from build123d import *

# Parameters (mm, degrees)
F0_R     = 1.5
F1_DEPTH = 3
F2_DEPTH = 7
F0_W     = 5
F0_H     = 56.2
F3_DEPTH = 23
F4_R     = 2.1
F5_DEPTH = 5
F6_R     = 5


with BuildPart() as f1:
    # F0 (on Top) → F1 (new body)
    with BuildSketch(Plane.XY):
        with BuildLine():
            Line((-39.5, 28.1), (-41.7, 28.1))
            ThreePointArc((-41.7, 28.1), (-42.4071067812, 27.8071067812), (-42.7, 27.1))
            Line((-42.7, 27.1), (-42.7, -27.1))
            ThreePointArc((-42.7, -27.1), (-42.4071067812, -27.8071067812), (-41.7, -28.1))
            Line((-41.7, -28.1), (-39.5, -28.1))
            Line((-39.5, -28.1), (39.5, -28.1))
            Line((39.5, -28.1), (41.7, -28.1))
            ThreePointArc((41.7, -28.1), (42.4071067812, -27.8071067812), (42.7, -27.1))
            Line((42.7, -27.1), (42.7, 27.1))
            ThreePointArc((42.7, 27.1), (42.4071067812, 27.8071067812), (41.7, 28.1))
            Line((41.7, 28.1), (39.5, 28.1))
            Line((39.5, 28.1), (-39.5, 28.1))
        make_face()
        with BuildLine():
            ThreePointArc((-36.4, -25), (-37.3079689783, -27.1920310217), (-39.5, -28.1))
            ThreePointArc((-39.5, -28.1), (-41.6920310217, -22.8079689783), (-36.4, -25))
        make_face(mode=Mode.SUBTRACT)
        with BuildLine():
            Line((27.5, -17), (-27.5, -17))
            ThreePointArc((-27.5, -17), (-31, -13.5), (-27.5, -10))
            Line((-27.5, -10), (27.5, -10))
            ThreePointArc((27.5, -10), (31, -13.5), (27.5, -17))
        make_face(mode=Mode.SUBTRACT)
        with BuildLine():
            ThreePointArc((42.6, -25), (41.6920310217, -27.1920310217), (39.5, -28.1))
            ThreePointArc((39.5, -28.1), (37.3079689783, -22.8079689783), (42.6, -25))
        make_face(mode=Mode.SUBTRACT)
        with BuildLine():
            ThreePointArc((-27.5, 10), (-31, 13.5), (-27.5, 17))
            Line((-27.5, 17), (27.5, 17))
            ThreePointArc((27.5, 17), (31, 13.5), (27.5, 10))
            Line((27.5, 10), (-27.5, 10))
        make_face(mode=Mode.SUBTRACT)
        with BuildLine():
            ThreePointArc((-36.4, 25), (-41.6920310217, 22.8079689783), (-39.5, 28.1))
            ThreePointArc((-39.5, 28.1), (-37.3079689783, 27.1920310217), (-36.4, 25))
        make_face(mode=Mode.SUBTRACT)
        with BuildLine():
            ThreePointArc((42.6, 25), (37.3079689783, 22.8079689783), (39.5, 28.1))
            ThreePointArc((39.5, 28.1), (41.6920310217, 27.1920310217), (42.6, 25))
        make_face(mode=Mode.SUBTRACT)
        with BuildLine():
            Line((45.7, 28.1), (41.7, 28.1))
            ThreePointArc((41.7, 28.1), (42.4071067812, 27.8071067812), (42.7, 27.1))
            Line((42.7, 27.1), (42.7, -27.1))
            ThreePointArc((42.7, -27.1), (42.4071067812, -27.8071067812), (41.7, -28.1))
            Line((41.7, -28.1), (45.7, -28.1))
            Line((45.7, -28.1), (45.7, 28.1))
        make_face()
        with BuildLine():
            ThreePointArc((-36.4, 25), (-37.3079689783, 27.1920310217), (-39.5, 28.1))
            ThreePointArc((-39.5, 28.1), (-41.6920310217, 22.8079689783), (-36.4, 25))
        make_face()
        with Locations((-39.5, 25)):
            Circle(F0_R, mode=Mode.SUBTRACT)
        with BuildLine():
            ThreePointArc((-36.4, -25), (-41.6920310217, -22.8079689783), (-39.5, -28.1))
            ThreePointArc((-39.5, -28.1), (-37.3079689783, -27.1920310217), (-36.4, -25))
        make_face()
        with Locations((-39.5, -25)):
            Circle(F0_R, mode=Mode.SUBTRACT)
        with BuildLine():
            ThreePointArc((42.6, -25), (37.3079689783, -22.8079689783), (39.5, -28.1))
            ThreePointArc((39.5, -28.1), (41.6920310217, -27.1920310217), (42.6, -25))
        make_face()
        with Locations((39.5, -25)):
            Circle(F0_R, mode=Mode.SUBTRACT)
        with BuildLine():
            ThreePointArc((42.6, 25), (41.6920310217, 27.1920310217), (39.5, 28.1))
            ThreePointArc((39.5, 28.1), (37.3079689783, 22.8079689783), (42.6, 25))
        make_face()
        with Locations((39.5, 25)):
            Circle(F0_R, mode=Mode.SUBTRACT)
        with Locations((-39.5, 25)):
            Circle(F0_R)
        with Locations((-39.5, -25)):
            Circle(F0_R)
        with Locations((39.5, -25)):
            Circle(F0_R)
        with Locations((39.5, 25)):
            Circle(F0_R)
    extrude(amount=F1_DEPTH)

    # F0 (on Top) → F2 (join)
    with BuildSketch(Plane.XY):
        with BuildLine():
            ThreePointArc((-36.4, 25), (-37.3079689783, 27.1920310217), (-39.5, 28.1))
            ThreePointArc((-39.5, 28.1), (-41.6920310217, 22.8079689783), (-36.4, 25))
        make_face()
        with Locations((-39.5, 25)):
            Circle(F0_R, mode=Mode.SUBTRACT)
        with BuildLine():
            ThreePointArc((-36.4, -25), (-41.6920310217, -22.8079689783), (-39.5, -28.1))
            ThreePointArc((-39.5, -28.1), (-37.3079689783, -27.1920310217), (-36.4, -25))
        make_face()
        with Locations((-39.5, -25)):
            Circle(F0_R, mode=Mode.SUBTRACT)
        with BuildLine():
            ThreePointArc((42.6, -25), (37.3079689783, -22.8079689783), (39.5, -28.1))
            ThreePointArc((39.5, -28.1), (41.6920310217, -27.1920310217), (42.6, -25))
        make_face()
        with Locations((39.5, -25)):
            Circle(F0_R, mode=Mode.SUBTRACT)
        with BuildLine():
            ThreePointArc((42.6, 25), (41.6920310217, 27.1920310217), (39.5, 28.1))
            ThreePointArc((39.5, 28.1), (37.3079689783, 22.8079689783), (42.6, 25))
        make_face()
        with Locations((39.5, 25)):
            Circle(F0_R, mode=Mode.SUBTRACT)
    extrude(amount=F2_DEPTH)

    # F0 (on Top) → F3 (join)
    with BuildSketch(Plane.XY):
        with Locations((48.2, 0)):
            Rectangle(F0_W, F0_H)
    extrude(amount=F3_DEPTH)

    # F4 (on face) → F5 (cut, through all)
    with BuildSketch(Plane.YZ.offset(50.7)):
        with Locations((-21, 13)):
            Circle(F4_R)
        with Locations((21, 13)):
            Circle(F4_R)
    extrude(amount=-F5_DEPTH, mode=Mode.SUBTRACT)

    # F6
    f6_edges = [f1.edges().sort_by_distance(p)[0] for p in [
        (48.2, 28.1, 23),
        (48.2, -28.1, 23),
    ]]
    fillet(f6_edges, radius=F6_R)


solid = f1.part
Can you work these out from the model? Positions are in its coordinate system, mm. A direction names the side the tool comes from. Coordinates: 2 decimals unless noted, no trailing zeros. Order: outer loops, then holes, each group sorted by start corner. A loop starts at its lowest first (then second) coordinate and runs counter-clockwise, first axis right, second up. Notation, with made-up numbers: M 41.5,8 L 65.5,8 A11 cw 65.5,17 Z; hole C -38.5,-15.5 d11. An arc over 180 degrees is marked long. Write item = value, one per line.
(1) Suppose I cut it at C-C on z = 16. Please give me the cut outline in (x, y), plus the area to 3 significant figures.
Results are:
outline = M 45.7,-28.1 L 50.7,-28.1 L 50.7,28.1 L 45.7,28.1 Z
area = 281 mm2
(2) For faces 1 (the face through (-38, -24, 7)), 2 (the face through (-40.61, -23.99, 4.97)), 3 (the face through (48, 0, 23)), 4 (the face through (-31, 13.4, 1.5)), 5 (the face through (48.235, -18.997, 13.631)), which set-ups out of +Z, -Z, +X, -X, +Y, -Y let a thin tool reach every point of the face, with its end or its side?
Results are:
face_1 = +Z, -X, +Y, -Y
face_2 = +Z
face_3 = +Z, +X, -X, +Y, -Y
face_4 = +Z, -Z
face_5 = +X, -X
(3) For pin 1 Ø1.5 at (x, y) = (-30.5, -21.5) entering from +Z; pin 2 Ø2.5 at (x, y) = (-40, -24.5) entering from +Z; pin 3 Ø5 at (y, z) = (18.5, 12.5) entering from -X, each with a flat end and sliding along its axis, tell me the tip position at first contact or that it passes through.
Results are:
pin_1 = 3
pin_2 = 7
pin_3 = 45.7
(4) I need wall thicknesses on line 1 along Y through (x, z) = (-39.5, 5.35); line 2 along X through (y, z) = (25, 3.9); line 3 along Z through (x, y) = (48, -21). Which ranges of each line are inside material? Lowest first, please. Write a range as [from, to].
Results are:
line_1 = [-28.1, -26.5], [-23.5, -21.9], [21.9, 23.5], [26.5, 28.1]
line_2 = [-42.6, -41], [-38, -36.4], [36.4, 38], [41, 42.6], [45.7, 50.7]
line_3 = [0, 10.9], [15.1, 23]
(5) If we mould it in two halves opening along X, with no side actions, what happens to faces 6 (the face through (31, 13.6, 1.5)), 7 (the face through (11, -28.1, 2))? For each: pulls with the +X half, pulls with the -X half, needs draft (parallel to the pull), parting line crosses it, or undercut.
Results are:
face_6 = undercut
face_7 = needs draft
(6) Suppose I cut it at A-A on x = -3.5. Please give me the cut outline in (y, z), plus the area to 3 significant figures.
Results are:
outline = M -28.1,0 L -17,0 L -17,3 L -28.1,3 Z; M -10,0 L 10,0 L 10,3 L -10,3 Z; M 17,0 L 28.1,0 L 28.1,3 L 17,3 Z
area = 127 mm2
(7) Suppose I cut it at D-D on x = -28.5. Please give me the cut outline in (y, z).
Results are:
outline = M -28.1,0 L -16.85,0 L -16.85,3 L -28.1,3 Z; M -10.15,0 L 10.15,0 L 10.15,3 L -10.15,3 Z; M 16.85,0 L 28.1,0 L 28.1,3 L 16.85,3 Z
(8) Suppose I cut it at B-B on y = 21. Please give me the cut outline in (x, z), plus the area to 3 significant figures.
Results are:
outline = M -42.7,0 L 50.7,0 L 50.7,10.9 L 45.7,10.9 L 45.7,3 L -42.7,3 Z; M 45.7,15.1 L 50.7,15.1 L 50.7,23 L 45.7,23 Z
area = 359 mm2
